Verification items for this drawing (mm, ordinates from the low corner). A direction names the side the tool comes from. Give positions to 0.01 mm unless a question says otherwise; leave off trailing zeros. Write each loop counter-clockwise with the first axis right and the second up, starting at its lowest first coordinate (ties: lowest second). Pieces come first, ordered by that corner, then holes. Notation, with made-up numbers: (5, 74.25) -> (56, 74.25) arc R33 cw to (56, 108.25) -> close; hole circle Ø10 at (-23.5, 45.25). An arc over 180 degrees is marked (long way). Use one line per item in the form item = value. Start each with the question number.
(1) Section check A-A, the plane z = 13.25. Record the cut outline in (x, y).
(2) Section check C-C, the plane y = 17. Record the cut outline in (x, z), plus the area to 3 significant figures.
(3) Scan lines: L1, parallel to X at y = 28, z = 13; L2, parallel to X at y = 26.5, z = 5; L3, parallel to Z at x = 14.25, y = 2.5. Record each from-to range of solid material in increasing order.
(4) Release check for a two-part mould opening along X. For the marked faces 1, 2 and 3 record: pulls with the +X half, pulls with the -X half, needs draft (parallel to the pull), parting line crosses it, or undercut.
(5) Section check B-B, the plane z = 5.5. Record the cut outline in (x, y), plus the area to 3 significant figures.
(6) Set-up check for the marked faces 4 and 5: record each of +Z, -Z, +X, -X, +Y, -Y from which the full face is reachable in a straight line by a thin tool's end or side.
(7) Depth check by flat-ended pin: pin 1 Ø1 at (x, y) = (4, 3.5) entering from -Z; pin 2 Ø0.6 at (x, y) = (19.5, 16.5) entering from +Z. Enter the tip coordinate at first touch or a pass-through.
(8) Section check D-D, the plane x = 18.25. Record the cut outline in (y, z), plus the area to 3 significant figures.
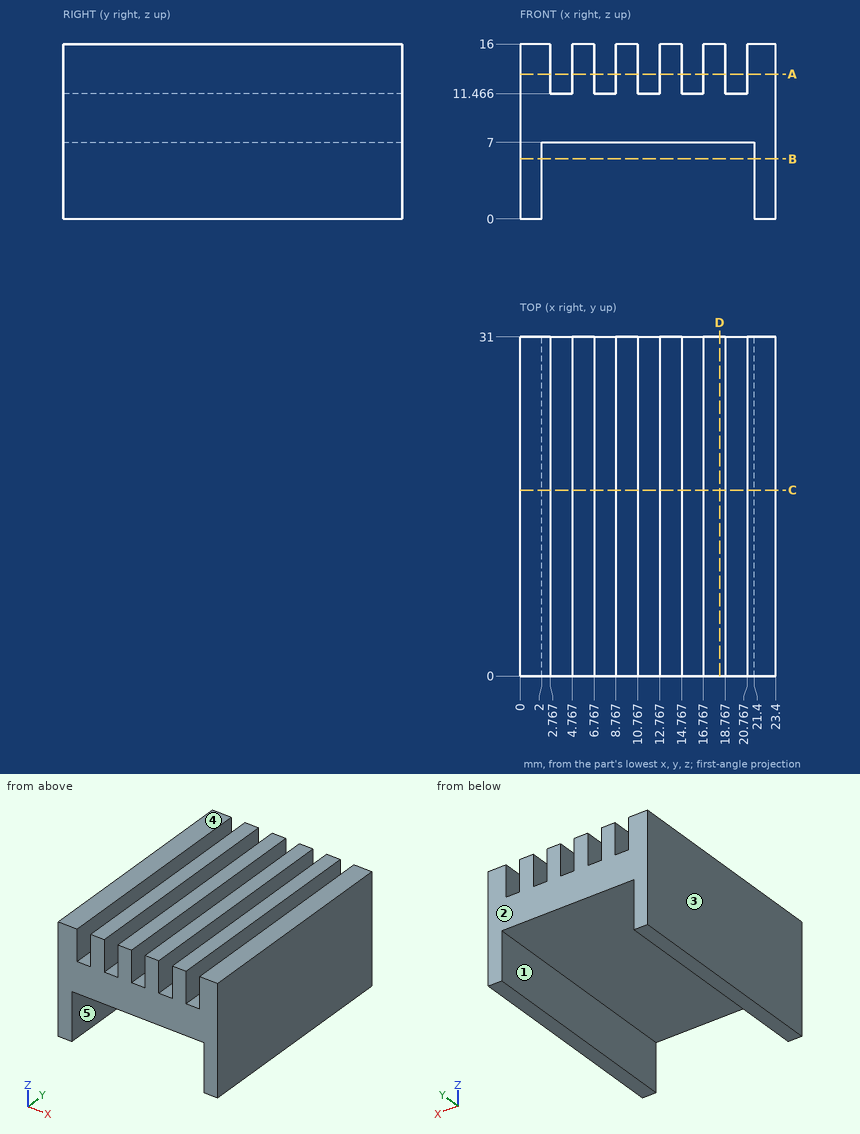
Completed:
q1.outline = (0, 0) -> (2.77, 0) -> (2.77, 31) -> (0, 31) -> close; (4.77, 0) -> (6.77, 0) -> (6.77, 31) -> (4.77, 31) -> close; (8.77, 0) -> (10.77, 0) -> (10.77, 31) -> (8.77, 31) -> close; (12.77, 0) -> (14.77, 0) -> (14.77, 31) -> (12.77, 31) -> close; (16.77, 0) -> (18.77, 0) -> (18.77, 31) -> (16.77, 31) -> close; (20.77, 0) -> (23.4, 0) -> (23.4, 31) -> (20.77, 31) -> close
q2.outline = (0, 0) -> (2, 0) -> (2, 7) -> (21.4, 7) -> (21.4, 0) -> (23.4, 0) -> (23.4, 16) -> (20.77, 16) -> (20.77, 11.47) -> (18.77, 11.47) -> (18.77, 16) -> (16.77, 16) -> (16.77, 11.47) -> (14.77, 11.47) -> (14.77, 16) -> (12.77, 16) -> (12.77, 11.47) -> (10.77, 11.47) -> (10.77, 16) -> (8.77, 16) -> (8.77, 11.47) -> (6.77, 11.47) -> (6.77, 16) -> (4.77, 16) -> (4.77, 11.47) -> (2.77, 11.47) -> (2.77, 16) -> (0, 16) -> close
q2.area = 193 mm²
q3.L1 = 0 to 2.77, 4.77 to 6.77, 8.77 to 10.77, 12.77 to 14.77, 16.77 to 18.77, 20.77 to 23.4
q3.L2 = 0 to 2, 21.4 to 23.4
q3.L3 = 7 to 16
q4.face_1 = undercut
q4.face_2 = needs draft
q4.face_3 = pulls with the -X half
q5.outline = (0, 0) -> (2, 0) -> (2, 31) -> (0, 31) -> close; (21.4, 0) -> (23.4, 0) -> (23.4, 31) -> (21.4, 31) -> close
q5.area = 124 mm²
q6.face_4 = +Z, +X, -X, +Y, -Y
q6.face_5 = -Z, +Y, -Y
q7.pin_1 = 7
q7.pin_2 = 11.47
q8.outline = (0, 7) -> (31, 7) -> (31, 16) -> (0, 16) -> close
q8.area = 279 mm²
